```python
from build123d import *

# Parameters (mm, degrees)
F0_W      = 30
F0_H      = 18
F1_DEPTH  = 2
F3_W      = 10
F3_H      = 18
F3_W_2    = 6
F3_H_2    = 14
F4_DEPTH  = 12
F6_W      = 6
F6_H      = 7.2452436302
F7_DEPTH  = 4
F9_W      = 10
F9_H      = 9
F10_DEPTH = 2


with BuildPart() as f1:
    # F0 (on Top) → F1 (new body)
    with BuildSketch(Plane.XY):
        Rectangle(F0_W, F0_H)
    extrude(amount=F1_DEPTH)

    # F3 (on offset) → F4 (join)
    with BuildSketch(Plane.XY.offset(2)):
        Rectangle(F3_W, F3_H)
        Rectangle(F3_W_2, F3_H_2, mode=Mode.SUBTRACT)
    extrude(amount=F4_DEPTH)

    # F6 (on offset) → F7 (cut)
    with BuildSketch(Plane(origin=(0, 9, 0), x_dir=(-1, 0, 0), z_dir=(0, 1, 0))):
        with Locations((0, 10.3773781849)):
            Rectangle(F6_W, F6_H)
    extrude(amount=-F7_DEPTH, mode=Mode.SUBTRACT)

    # F9 (on offset) → F10 (join)
    with BuildSketch(Plane.XY.offset(14)):
        with Locations((0, -4.5)):
            Rectangle(F9_W, F9_H)
    extrude(amount=F10_DEPTH)


solid = f1.part
```
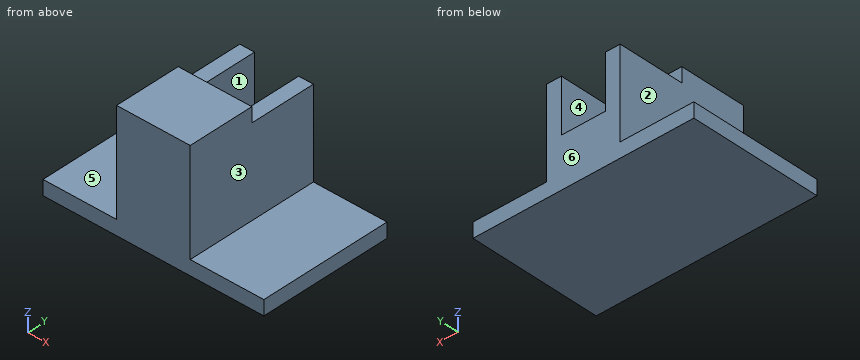
The listing builds one solid part. Answer for the finished solid, in the listing's coordinates (mm). Face numbers are marked on the shaded views. A direction names the side the tool comes from. Coordinates: 2 decimals unless noted, no trailing zeros. Write each loop counter-clockwise with the first axis right and the second up, starting at its lowest first coordinate (ties: lowest second). Pieces come first, ordered by that corner, then holes. Notation, with made-up numbers: M 63,10.5 L 104,10.5 A18 cw 104,42.5 Z; hole C -21,35.25 d1. An arc over 180 degrees is marked long. Use a Markdown table: item, result. Add a question column.
1. For a pull along Y with two mould halves and no side action, classify the marked faces 4, 5 and 6 as +Y half, -Y half, draft (parallel to the pull), parting line (faces both ways), or undercut.
2. Section C-C (x = 1.25) is taken. Give the vertices of the cut face in (y, z), plus the area to 3 significant figures.
3. Which of the six approach directions +Z, -Z, +X, -X, +Y, -Y give full straight-line access (tool end or side, diameter ignored) to the marked faces 1, 2 and 3?
4. Straight lines are drawn through the part: line 1 along Z through (x, y) = (0.5, -0.5); line 2 along X through (y, z) = (-0.5, 12.75); line 3 along Z through (x, y) = (-3.75, 1). For each, find the intervals that lie inside material, in ascending order. Write a range as [from, to].
5. Section B-B (z = 5.25) is taken. Give the vertices of the cut face in (x, y), plus the area to 3 significant figures.
6. Section D-D (y = 2) is taken. Give the vertices of the cut face in (x, z).
7. Given P1, Ø4, axis at y = -1, z = 11, coming from the -X side; P2, Ø4, axis at y = 7, z = 7.5, coming from the +X side; P3, Ø3, axis at x = -10.5, y = 2.5, coming from the +Z side; P4, Ø4, axis at x = 8, z = 5, coming from the -Y side, each flat-ended and moving along its own axis, determine where each tip first touches the part or whether it passes through.
8. Section A-A (y = -3.5) is taken. Give the vertices of the cut face in (x, z), plus the area to 3 significant figures.
Data:
| question | item | result |
|---|---|---|
| 1 | face 4 | undercut |
| 1 | face 5 | draft |
| 1 | face 6 | +Y half |
| 2 | outline | M -9,0 L 9,0 L 9,6.75 L 7,6.75 L 7,2 L -7,2 L -7,14 L 0,14 L 0,16 L -9,16 Z |
| 2 | area | 87.5 mm2 |
| 3 | face 1 | none |
| 3 | face 2 | +Z, -X, +Y, -Y |
| 3 | face 3 | +Z, +X, +Y, -Y |
| 4 | line 1 | z = [0, 2], [14, 16] |
| 4 | line 2 | x = [-5, -3], [3, 5] |
| 4 | line 3 | z = [0, 14] |
| 5 | outline | M -5,-9 L 5,-9 L 5,9 L -5,9 Z; hole M -3,-7 L 3,-7 L 3,7 L -3,7 Z |
| 5 | area | 96.0 mm2 |
| 6 | outline | M -15,0 L 15,0 L 15,2 L 5,2 L 5,14 L 3,14 L 3,2 L -3,2 L -3,14 L -5,14 L -5,2 L -15,2 Z |
| 7 | P1 | stops at x = -5 |
| 7 | P2 | stops at x = 5 |
| 7 | P3 | stops at z = 2 |
| 7 | P4 | passes through |
| 8 | outline | M -15,0 L 15,0 L 15,2 L 5,2 L 5,16 L -5,16 L -5,2 L -15,2 Z; hole M -3,2 L 3,2 L 3,14 L -3,14 Z |
| 8 | area | 128 mm2 |
